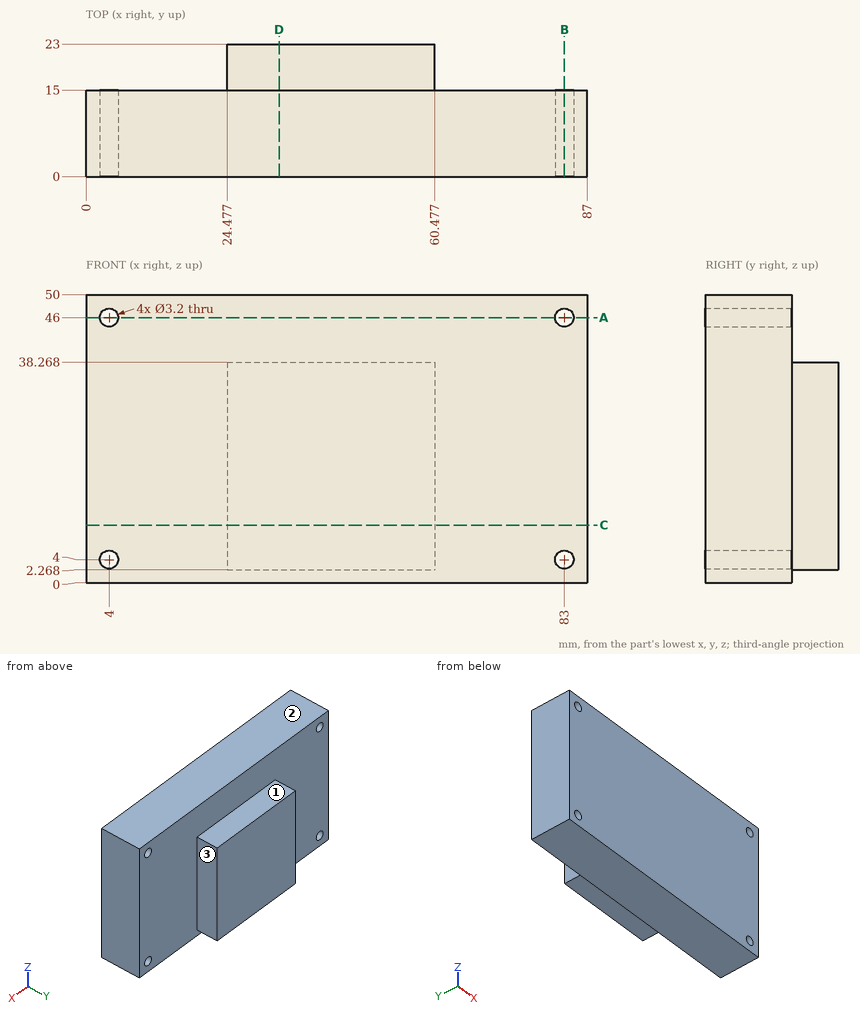
Design review of the part shown in the three views and the two pictorial views. Dimensions are in mm from the part's minimum x, y and z. A direction names the side the tool comes from. Round coordinates to 2 decimals unless told otherwise and drop trailing zeros. Order: outer loops, then holes, each group sorted by start corner. A loop starts at its lowest first (then second) coordinate and runs counter-clockwise, first axis right, second up. Notation, with made-up numbers: (6.5, 50) -> (19.5, 50) arc R33 cw to (19.5, 79) -> close; hole circle Ø9 at (13, 46). An arc over 180 degrees is marked (long way). Write item = value, one per line. Start each with the question number.
1) Tool access review of the marked faces 1, 2 and 3: name each direction out of +Z, -Z, +X, -X, +Y, -Y from which nothing blocks a thin tool from reaching the whole face with its end or side.
2) Insertion check: pin 1 (5 mm diameter, centred on x = 83, z = 4, fed in from +Y); pin 2 (8 mm diameter, centred on x = 44, y = 18.5, fed in from -Z); pin 3 (5 mm diameter, centred on y = 19, z = 38, fed in from +X); pin 4 (6.5 mm diameter, centred on x = 42, y = 19.5, fed in from +Z). Each pin has a flat end and moves straight along its axis. Give the tip position at first contact, or say it passes through.
3) To check wall thickness, follow line 1 (X direction, y = 3.75, z = 4); line 2 (Z direction, x = 83, y = 11.25); line 3 (Y direction, x = 77, z = 18.5). State the ranges of each line that lie inside material, in increasing order. Write a range as from..to.
4) Take a section at D-D on x = 33.5. State the section outline as (y, z) points.
5) Take a section at B-B on x = 83. State the section outline as (y, z) points, plus the area to 3 significant figures.
6) Take a section at A-A on z = 46. State the section outline as (x, y) points.
7) Take a section at C-C on z = 10. State the section outline as (x, y) points.
Verdict:
q1.face_1 = +Z, +X, -X, +Y
q1.face_2 = +Z, +X, -X, +Y, -Y
q1.face_3 = +Z, -Z, +X, +Y
q2.pin_1 = 15
q2.pin_2 = 0
q2.pin_3 = 60.48
q2.pin_4 = 38.27
q3.line_1 = 0..2.4, 5.6..81.4, 84.6..87
q3.line_2 = 0..2.4, 5.6..44.4, 47.6..50
q3.line_3 = 0..15
q4.outline = (0, 0) -> (15, 0) -> (15, 2.27) -> (23, 2.27) -> (23, 38.27) -> (15, 38.27) -> (15, 50) -> (0, 50) -> close
q5.outline = (0, 0) -> (15, 0) -> (15, 2.4) -> (0, 2.4) -> close; (0, 5.6) -> (15, 5.6) -> (15, 44.4) -> (0, 44.4) -> close; (0, 47.6) -> (15, 47.6) -> (15, 50) -> (0, 50) -> close
q5.area = 654 mm2
q6.outline = (0, 0) -> (2.4, 0) -> (2.4, 15) -> (0, 15) -> close; (5.6, 0) -> (81.4, 0) -> (81.4, 15) -> (5.6, 15) -> close; (84.6, 0) -> (87, 0) -> (87, 15) -> (84.6, 15) -> close
q7.outline = (0, 0) -> (87, 0) -> (87, 15) -> (60.48, 15) -> (60.48, 23) -> (24.48, 23) -> (24.48, 15) -> (0, 15) -> close
